Source: CAD feature listing. Evaluate the final solid. Frame: model axes, mm. A direction names the side the tool comes from. Give positions to 0.01 mm unless a question says otherwise; leave off trailing zeros. Loops run counter-clockwise (first coordinate to the right, second up) from the corner with the lowest first, then second, coordinate; pieces in that order, holes last. Notation, with made-up numbers: (88, 57.25) -> (124, 57.25) arc R26 cw to (124, 77.25) -> close; hole circle Ø8 at (-33.75, 24). An arc over 180 degrees is marked (long way). Return JSON: item names as keys, results as strings. Group by question number.
(1) Pin query (flat end, axial travel): pin 1 (0.5 mm diameter, centred on y = 2.5, z = -10, fed in from +X); pin 2 (0.8 mm diameter, centred on y = 14, z = -10, fed in from -X); pin 3 (1 mm diameter, centred on x = 5, y = 11, fed in from +Z). Return the tip coordinate at first contact, or that it passes through.
(2) Ray query, line 1 (Y direction, x = 5.5, z = 9.25); line 2 (Y direction, x = 8.5, z = -4.75); line 3 (Y direction, x = 6.75, z = 4.5). Return the intervals inside material, ascending. Write a range as from..to.
(3) Access query for faces 1 (the face through (-3.905, 24.351, -0.867)), 2 (the face through (0, 2, -10)), 3 (the face through (0, 27.9, 0)). Directions: +Z, -Z, +X, -X, +Y, -Y. A direction counts if a zero-diameter tool reaches every point of the face in a straight line with its end or side. Return the directions, or none.
(4) Cut plane C-C on y = 25.5. Return loops of the section in (x, z), then the cut area to 3 significant figures.
(5) Draft query along Y for faces 4 (the face through (-3.92, 20.9, -1.42)), 5 (the face through (0, 14, -10)), 6 (the face through (1.802, 19.886, 5.723)), 7 (the face through (2.873, 15.665, 9.123)). Return one class per face: released by +Y, released by -Y, zero draft, split by the parting line, or undercut.
(6) Cut plane A-A on x = 10.25. Give the number of separate pieces and of enclosed holes in the cut face, then the cut area to 3 significant figures.
```python
from build123d import *
from build123d.topology import SkipClean

# Parameters (mm, degrees)
SKETCH_1_R      = 9.4
EXTRUDE_1_DEPTH = 15.5
SKETCH_3_R      = 6
EXTRUDE_2_DEPTH = 2
SKETCH_4_R      = 4
EXTRUDE_3_DEPTH = 7
SWEEP_1_PITCH   = 4


with BuildPart() as part:
    # 草图1 → 凸台-拉伸1 (new body)
    with BuildSketch(Plane(origin=(0, 0, 0), x_dir=(1, 0, 0), z_dir=(0, 1, 0))):
        with Locations(Location((0, 0, 0), (0, 0, 270))):
            Circle(SKETCH_1_R)
    extrude(amount=EXTRUDE_1_DEPTH)

    # 草图2 → 旋转1 (revolve)
    with BuildSketch(Plane.XY, mode=Mode.PRIVATE) as revolve_1_sk:
        Polygon((0, 18.9), (12.8, 18.9), (9.4, 15.5), (0, 15.5), align=None)
    revolve(revolve_1_sk.sketch.rotate(Axis((0, 15.5, 0), (0, 1, 0)), 270), axis=Axis((0, 15.5, 0), (0, 1, 0)))

    # 草图3 → 凸台-拉伸2 (add)
    with BuildSketch(Plane(origin=(0, 18.9, 0), x_dir=(1, 0, 0), z_dir=(0, 1, 0))):
        with Locations(Location((0, 0, 0), (0, 0, 270))):
            Circle(SKETCH_3_R)
    extrude(amount=EXTRUDE_2_DEPTH)

    # 草图4 → 凸台-拉伸3 (add)
    with BuildSketch(Plane(origin=(0, 20.9, 0), x_dir=(1, 0, 0), z_dir=(0, 1, 0))):
        with Locations(Location((0, 0, 0), (0, 0, 270))):
            Circle(SKETCH_4_R)
    extrude(amount=EXTRUDE_3_DEPTH)

    # 扫描1: the profile of 草图8 profile screwed along a right-hand helix of 3 turns, 12 arcs to a turn; built about Z, then put on its axis
    with SkipClean():  # the faces are left unmerged after this step: merging them gives an invalid solid
        sweep_1_z = Axis((0, 0, 0), (0, 0, 1))
        sweep_1_corners = [(9.3997, 0, 1.7503), (9.3997, 0, -1.7503), (10.9, 0, -0.25), (10.9, 0, 0.25)]
        with BuildLine(mode=Mode.PRIVATE) as sweep_1_profile:
            Line(sweep_1_corners[0], sweep_1_corners[1])
            Line(sweep_1_corners[1], sweep_1_corners[2])
            Line(sweep_1_corners[2], sweep_1_corners[3])
            Line(sweep_1_corners[3], sweep_1_corners[0])
        sweep_1_cap = Face(sweep_1_profile.wire())
        sweep_1_turn_angles = [0, 15, 30, 45, 60, 75, 90, 105, 120, 135, 150, 165, 180, 195, 210, 225, 240, 255, 270, 285, 300, 315, 330, 345, 360]
        sweep_1_turn_weights = [1, 0.9659258262890683, 1, 0.9659258262890683, 1, 0.9659258262890683, 1, 0.9659258262890683, 1, 0.9659258262890683, 1, 0.9659258262890683, 1, 0.9659258262890683, 1, 0.9659258262890683, 1, 0.9659258262890683, 1, 0.9659258262890683, 1, 0.9659258262890683, 1, 0.9659258262890683, 1]
        sweep_1_turn_rails = [Edge.make_bspline([Vector(p[0], p[1], 0).rotate(sweep_1_z, sweep_1_turn_angles[k]) / sweep_1_turn_weights[k] + Vector(0, 0, p[2] + SWEEP_1_PITCH * sweep_1_turn_angles[k] / 360) for k in range(25)], [0, 0, 0, 1, 1, 2, 2, 3, 3, 4, 4, 5, 5, 6, 6, 7, 7, 8, 8, 9, 9, 10, 10, 11, 11, 12, 12, 12], 2, sweep_1_turn_weights) for p in sweep_1_corners]
        sweep_1_turn_sides = [Face.make_surface_from_curves(sweep_1_turn_rails[p[0]], sweep_1_turn_rails[p[1]]) for p in [(0, 1), (1, 2), (2, 3), (3, 0)]]
        sweep_1 = Plane(origin=(0, 1.75, 0), x_dir=(0, 0, -1), z_dir=(0, 1, 0)) * Solid(Shell([*[p.moved(Location((0, 0, SWEEP_1_PITCH * i))) for i in range(3) for p in sweep_1_turn_sides], sweep_1_cap, sweep_1_cap.rotate(sweep_1_z, 1080).moved(Location((0, 0, SWEEP_1_PITCH * 1080 / 360)))]))
        add(sweep_1)


solid = part.part
```
Answers:
{
 "1": {"pin 1": "x = 0", "pin 2": "x = 0", "pin 3": "z = 9.4"},
 "2": {"line 1": "3.7..4.48, 7.7..8.48, 11.7..12.48, 16.86..18.9", "line 2": "3.66..6.49, 7.66..10.49, 11.66..14.49, 15.84..18.9", "line 3": "0..18.9"},
 "3": {"face 1": "+Y", "face 2": "-Z, +X, -Y", "face 3": "+Z, -Z, +X, -X, +Y"},
 "4": {"outline": "circle Ø8 at (0, 0)", "area": "50.3 mm²"},
 "5": {"face 4": "released by +Y", "face 5": "undercut", "face 6": "zero draft", "face 7": "undercut"},
 "6": {"separate pieces": "4", "enclosed holes": "0", "area": "55.8 mm²"}
}
